Input: part model. Units: mm. Frame: model coordinates. Face numbers are marked on the shaded views. A direction names the side the tool comes from. Give positions to 0.01 mm unless a question says otherwise; leave off trailing zeros. Loops run counter-clockwise (first coordinate to the right, second up) from the corner with the lowest first, then second, coordinate; pieces in that order, holes last. Notation, with made-up numbers: M -14.5,48 L 18.5,48 A13 ccw 18.5,65 Z; hole C -33.75,25 d11. An arc over 180 degrees is marked long. Return JSON: item names as keys, results as strings. Group by question number.
```python
from build123d import *

# Parameters (mm, degrees)
F0_R     = 1.5
F1_DEPTH = 18
F2_R     = 2.75
F3_DEPTH = 3
F5_DEPTH = 1.3
F6_SIZE  = 0.2


with BuildPart() as f1:
    # F0 (on Front) → F1 (new body)
    with BuildSketch(Plane.XZ):
        Circle(F0_R)
    extrude(amount=F1_DEPTH)

    # F2 (on face) → F3 (join)
    with BuildSketch(Plane.XZ.offset(18)):
        Circle(F2_R)
    extrude(amount=F3_DEPTH)

    # F4 (on face) → F5 (cut)
    with BuildSketch(Plane.XZ.offset(21)):
        Polygon((0.2100819211, -1.428005224), (1.3417297613, -0.5320663314), (1.1316478402, 0.8959388926), (-0.2100819211, 1.428005224), (-1.3417297613, 0.5320663314), (-1.1316478402, -0.8959388926), align=None)
    extrude(amount=-F5_DEPTH, mode=Mode.SUBTRACT)

    # F6
    f6_edges = [f1.edges().sort_by_distance(p)[0] for p in [
        (-2.75, -21, 0),
        (-2.75, -18, 0),
        (-1.5, 0, 0),
        (-1.236689, -21, -0.181936),
        (-0.460783, -21, -1.161972),
        (0.775906, -21, -0.980036),
        (1.236689, -21, 0.181936),
        (0.460783, -21, 1.161972),
        (-0.775906, -21, 0.980036),
    ]]
    chamfer(f6_edges, length=F6_SIZE)


solid = f1.part
```
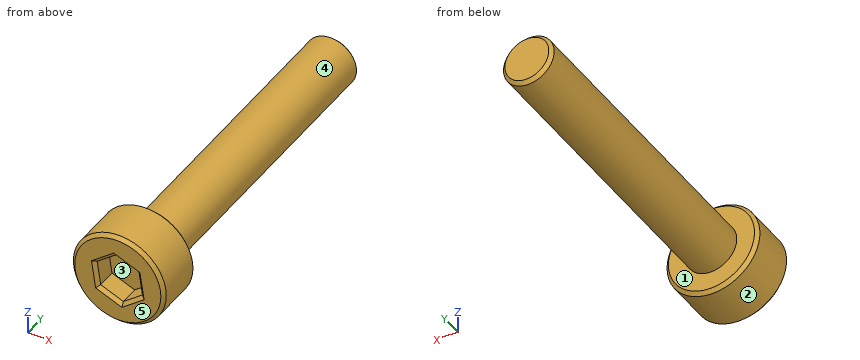
Item 1: Material intervals for line 1 (X direction, y = -18.5, z = 0.15); line 2 (Z direction, x = 0.1, y = -3.5); line 3 (Y direction, x = 0.8, z = -1.8), sorted ascending. Write a range as from..to.
Item 2: Section C-C, the plane x = 0. Return loops of the section in (y, z).
Item 3: Section B-B, the plane y = -6. Return loops of the section in (x, z).
Item 4: Reachability of the marked faces 1 and 2 from +Z, -Z, +X, -X, +Y, -Y: full face, straight path, thin tool, end or side. Return the list, or none.
Item 5: First-contact query: pin 1 Ø2 at (x, z) = (0.5, 0.5) entering from -Y; pin 2 Ø1.5 at (x, y) = (1.5, -16.5) entering from +Z; pin 3 Ø1 at (y, z) = (-4, 1) entering from +X; pin 4 Ø1 at (x, y) = (0, -13.5) entering from +Z. Flat tips, straight axial feed; report the tip coordinate or a pass-through.
Item 6: Section A-A, the plane z = 0. Return loops of the section in (x, y), then the cut area to 3 significant figures.
Item 7: Pull-direction query (X, two-part tool) for the marked faces 3, 4 and 5; classes: pulls with the +X half, pulls with the -X half, needs draft (parallel to the pull), parting line crosses it, or undercut.
Answer below:
{
 "1": {"line 1": "-2.75..2.75", "line 2": "-1.5..1.5", "line 3": "-21..-18"},
 "2": {"outline": "M -21,-2.55 L -20.8,-2.75 L -18.2,-2.75 L -18,-2.55 L -18,-1.5 L -0.2,-1.5 L 0,-1.3 L 0,1.3 L -0.2,1.5 L -18,1.5 L -18,2.55 L -18.2,2.75 L -20.8,2.75 L -21,2.55 L -21,1.56 L -20.8,1.34 L -19.7,1.34 L -19.7,-1.34 L -20.8,-1.34 L -21,-1.56 Z"},
 "3": {"outline": "C 0,0 d3"},
 "4": {"face 1": "+Y", "face 2": "+Y, -Y"},
 "5": {"pin 1": "y = -21", "pin 2": "z = 1.3", "pin 3": "x = 1.41", "pin 4": "z = 1.5"},
 "6": {"outline": "M -2.75,-20.8 L -2.55,-21 L -1.47,-21 L -1.26,-20.8 L -1.26,-19.7 L 1.26,-19.7 L 1.26,-20.8 L 1.47,-21 L 2.55,-21 L 2.75,-20.8 L 2.75,-18.2 L 2.55,-18 L 1.5,-18 L 1.5,-0.2 L 1.3,0 L -1.3,0 L -1.5,-0.2 L -1.5,-18 L -2.55,-18 L -2.75,-18.2 Z", "area": "67.1 mm^2"},
 "7": {"face 3": "undercut", "face 4": "parting line crosses it", "face 5": "needs draft"}
}
